```python
from build123d import *

# Parameters (mm, degrees)
CUT_EXTRUDE1_DEPTH = 2


with BuildPart() as part:
    # Sketch1 → Base-Revolve (revolve)
    with BuildSketch(Plane.XY, mode=Mode.PRIVATE) as base_revolve_sk:
        with BuildLine():
            Line((0, -6.334936491), (0, 2.5))
            Line((0, 2.5), (1.75, 2.5))
            ThreePointArc((1.75, 2.5), (2.103553391, 2.353553391), (2.25, 2))
            Line((2.25, 2), (2.25, 0))
            Line((2.25, 0), (1.25, 0))
            Line((1.25, 0), (1.25, -6))
            Line((1.25, -6), (0, -6.334936491))
        make_face()
    revolve(base_revolve_sk.sketch.rotate(Axis((0, 2.5, 0), (0, 1, 0)), 90), axis=Axis((0, 2.5, 0), (0, 1, 0)))  # turned: the seam where the file's is

    # Sketch2 → Cut-Extrude1 (cut)
    with BuildSketch(Plane(origin=(0, 2.5, 0), x_dir=(-1, 0, 0), z_dir=(0, 1, 0))):
        Polygon((-1.154700538, 0), (-0.577350269, -1), (0.577350269, -1), (1.154700538, 0), (0.577350269, 1), (-0.577350269, 1), align=None)
    extrude(amount=-CUT_EXTRUDE1_DEPTH, mode=Mode.SUBTRACT)


solid = part.part
```
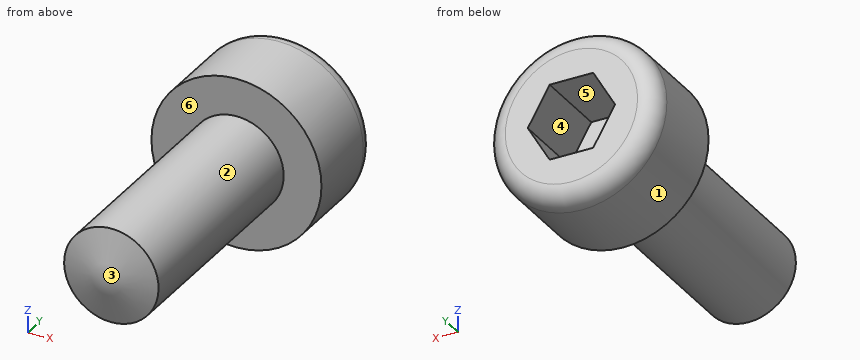
Geometry: final body of the model. Coordinates: model frame, mm. Face numbers are marked on the shaded views. A direction names the side the tool comes from. Give positions to 0.01 mm unless a question says otherwise; leave off trailing zeros. Write each loop counter-clockwise with the first axis right and the second up, starting at its lowest first coordinate (ties: lowest second). Pieces come first, ordered by that corner, then holes.
1. Pin query (flat end, axial travel): P1, Ø1.5, axis at x = -0.5, y = -2.5, coming from the -Z side; P2, Ø1.5, axis at x = 0, z = 1.5, coming from the -Y side. Return the tip coordinate at first contact, or that it passes through.
2. Reachability of the marked faces 1 and 2 from +Z, -Z, +X, -X, +Y, -Y: full face, straight path, thin tool, end or side. Return the list, or none.
3. Section query A-A, the plane y = -4.5. Return loops of the section in (x, z), then the cut area to 3 significant figures.
4. Line query: probe 1 along Y at (x, z) = (0.05, 1.6); probe 2 along Z at (x, y) = (0.65, -3.75); probe 3 along X at (y, z) = (1, -1.75). Output: solid intervals per line, ascending.
5. Draft query along Z for the marked faces 3, 4, 5 and 6. Return one class per face: released by +Z, released by -Z, zero draft, split by the parting line, or undercut.
Computed:
1. P1: stops at z = -1.25
1. P2: stops at y = -6.13
2. face 1: +Y, -Y
2. face 2: -Y
3. outline: circle Ø2.5 at (0, 0)
3. area: 4.91 mm2
4. probe 1: y = 0 to 2.5
4. probe 2: z = -1.07 to 1.07
4. probe 3: x = -1.41 to 1.41
5. face 3: split by the parting line
5. face 4: undercut
5. face 5: undercut
5. face 6: zero draft
